Build history of the part. All positions in model axes, mm. A direction names the side the tool comes from. Round coordinates to 2 decimals unless told otherwise and drop trailing zeros. Write each loop counter-clockwise with the first axis right and the second up, starting at its lowest first coordinate (ties: lowest second). Pieces come first, ordered by that corner, then holes. Notation, with made-up numbers: (47.25, 19) -> (52.25, 19) arc R22 cw to (52.25, 34) -> close; hole circle Ø4 at (18, -36.5). An arc over 180 degrees is marked (long way). One line per question, with ' | ' between items.
from build123d import *

# Parameters (mm, degrees)
SKETCH5_R                = 34
SKETCH5_R_2              = 19
BOSS_EXTRUDE1_DEPTH      = 4
SKETCH8_R                = 1.75
CUT_EXTRUDE3_DEPTH       = 5
SKETCH27_R               = 1.75
CUT_EXTRUDE9_DEPTH       = 5
SKETCH28_R               = 4.5
SKETCH28_R_2             = 1.75
CUT_EXTRUDE10_DEPTH      = 10
FILLET1_R                = 3
CIRPATTERN1_COUNT        = 4
FILLET1_OF_CIRPATTERN1_R = 3
SKETCH32_R               = 4
CUT_EXTRUDE11_DEPTH      = 10
FILLET2_R                = 2


with BuildPart() as part:
    # Sketch5 → Boss-Extrude1 (new body)
    with BuildSketch(Plane.XY):
        Circle(SKETCH5_R)
        Circle(SKETCH5_R_2, mode=Mode.SUBTRACT)
    extrude(amount=-BOSS_EXTRUDE1_DEPTH)

    # Sketch8 → Cut-Extrude3 (cut)
    with BuildSketch(Plane.XY):
        with Locations((20.859650045, 20.859650045)):
            Circle(SKETCH8_R)
        with Locations((-20.859650045, 20.859650045)):
            Circle(SKETCH8_R)
        with Locations((-20.859650045, -20.859650045)):
            Circle(SKETCH8_R)
        with Locations((20.859650045, -20.859650045)):
            Circle(SKETCH8_R)
    extrude(amount=-CUT_EXTRUDE3_DEPTH, mode=Mode.SUBTRACT)

    # Sketch27 → Cut-Extrude9 (cut)
    with BuildSketch(Plane.XY):
        with Locations((0, 29.5)):
            Circle(SKETCH27_R)
        with Locations((29.5, 0)):
            Circle(SKETCH27_R)
        with Locations((0, -29.5)):
            Circle(SKETCH27_R)
        with Locations((-29.5, 0)):
            Circle(SKETCH27_R)
    extrude(amount=-CUT_EXTRUDE9_DEPTH, mode=Mode.SUBTRACT)

    # Sketch28 → Cut-Extrude10 (cut)
    # profile 1 of 4: a face of its own
    with BuildSketch(Plane.XY):
        with BuildLine():
            Line((-4.5, 40.049875312), (-4.5, 33.700890196))
            ThreePointArc((-4.5, 33.700890196), (-2.254964893, 33.925140137), (0, 34))
            ThreePointArc((0, 34), (2.254964893, 33.925140137), (4.5, 33.700890196))
            Line((4.5, 33.700890196), (4.5, 40.049875312))
            Line((4.5, 40.049875312), (-4.5, 40.049875312))
        make_face()
    # profile 2 of 4: a face of its own
    with BuildSketch(Plane.XY):
        with BuildLine():
            Line((-4.5, 33.700890196), (-4.5, 29.5))
            ThreePointArc((-4.5, 29.5), (-3.181980515, 32.681980515), (0, 34))
            ThreePointArc((0, 34), (-2.254964893, 33.925140137), (-4.5, 33.700890196))
        make_face()
    # profile 3 of 4: a face of its own
    with BuildSketch(Plane.XY):
        with BuildLine():
            ThreePointArc((0, 34), (3.181980515, 32.681980515), (4.5, 29.5))
            Line((4.5, 29.5), (4.5, 33.700890196))
            ThreePointArc((4.5, 33.700890196), (2.254964893, 33.925140137), (0, 34))
        make_face()
    # profile 4 of 4: a face of its own
    with BuildSketch(Plane.XY):
        with Locations((0, 29.5)):
            Circle(SKETCH28_R)
        with Locations((0, 29.5)):
            Circle(SKETCH28_R_2, mode=Mode.SUBTRACT)
    cut_extrude10 = extrude(amount=-CUT_EXTRUDE10_DEPTH, mode=Mode.SUBTRACT)

    # Fillet1
    fillet1_edges = [part.edges().sort_by_distance(p)[0] for p in [
        (-4.5, 33.700890196, -2),
        (4.5, 33.700890196, -2),
    ]]
    fillet(fillet1_edges, radius=FILLET1_R)

    # CirPattern1: Cut-Extrude10 ×4 about axis
    cirpattern1_axis = Axis((0, 0, 0), (0, 0, 1))
    for i in range(1, CIRPATTERN1_COUNT):
        add(cut_extrude10.rotate(cirpattern1_axis, i * 360 / CIRPATTERN1_COUNT), mode=Mode.SUBTRACT)

    # Fillet1 of CirPattern1
    fillet1_of_cirpattern1_edges = [part.edges().sort_by_distance(p)[0] for p in [
        (-33.700890196, -4.5, -2),
        (-33.700890196, 4.5, -2),
        (4.5, -33.700890196, -2),
        (-4.5, -33.700890196, -2),
        (33.700890196, 4.5, -2),
        (33.700890196, -4.5, -2),
    ]]
    fillet(fillet1_of_cirpattern1_edges, radius=FILLET1_OF_CIRPATTERN1_R)

    # Sketch32 → Cut-Extrude11 (cut)
    with BuildSketch(Plane.XY):
        with Locations((-16.524893724, 9.376987118)):
            Circle(SKETCH32_R)
        with Locations((16.383155917, 9.622484201)):
            Circle(SKETCH32_R)
        with Locations((0.141737807, -18.999471319)):
            Circle(SKETCH32_R)
    extrude(amount=-CUT_EXTRUDE11_DEPTH, mode=Mode.SUBTRACT)

    # Fillet2
    fillet2_edges = [part.edges().sort_by_distance(p)[0] for p in [
        (-3.83907012, -18.608104165, -2),
        (4.116263726, -18.548756641, -2),
        (18.034625983, 5.979319831, -2),
        (14.005562597, 12.839167276, -2),
        (-14.195555863, 12.628784333, -2),
        (-18.121826323, 5.709589366, -2),
    ]]
    fillet(fillet2_edges, radius=FILLET2_R)


solid = part.part
(1) Drop flat-ended pins along their axis: pin 1 (1 mm diameter, centred on x = 21.5, z = -2.5, fed in from +Y); pin 2 (0.6 mm diameter, centred on y = -30, z = -1.5, fed in from -X); pin 3 (1 mm diameter, centred on y = -6.5, z = -3, fed in from -X). Give the stop position or say it passes through.
Calculated:
pin 1: y = 26.74 | pin 2: x = -16.55 | pin 3: x = -33.04
(2) 3-axis set-ups, long thin cutter, end or side, ignore diameter. For faces 1 (the cylindrical face through (5.683, 32.466, -2.028)), 2 (the cylindrical face through (16.424, -9.553, -1.972)): which of +Z, -Z, +X, -X, +Y, -Y reach the whole face in a straight line?
Calculated:
face 1: +Z, -Z, +Y | face 2: +Z, -Z
(3) Slice it at C-C (z = -2.3). State how many separate pieces and enclosed holes the cut face has, then the cut area to 3 significant figures.
Calculated:
separate pieces: 1 | enclosed holes: 5 | area: 2,070 mm2
(4) Wall check: line 1 (Y direction, x = -21, z = -2.2); line 2 (X direction, y = 0, z = -3.65); line 3 (Y direction, x = -22, z = -3.25). Give the ranges that are in metal, low to high. Write a range as from..to.
Calculated:
line 1: -26.74..-22.6, -19.12..19.12, 22.6..26.74 | line 2: -25..-19, 19..25 | line 3: -25.92..-22.19, -19.53..19.53, 22.19..25.92
(5) Slice it at A-A (y = 0). Write the cut outline in (x, z), then the cut area to 3 significant figures.
Calculated:
outline: (-25, -4) -> (-19, -4) -> (-19, 0) -> (-25, 0) -> close; (19, -4) -> (25, -4) -> (25, 0) -> (19, 0) -> close | area: 48.0 mm2
(6) Slice it at B-B (x = 0). Write the cut outline in (y, z).
Calculated:
outline: (-25, -4) -> (-23, -4) -> (-23, 0) -> (-25, 0) -> close; (19, -4) -> (25, -4) -> (25, 0) -> (19, 0) -> close
(7) Mould opens along Y. For faces 3 (the cylindrical face through (25, 0, -2)), 4 (the flat face through (-15, 15, 0)), 5 (the cylindrical face through (5.683, -32.466, -2.028)) say: pulls with the +Y half, pulls with the -Y half, needs draft (parallel to the pull), parting line crosses it, or undercut.
Calculated:
face 3: undercut | face 4: needs draft | face 5: pulls with the -Y half
